```python
from build123d import *

# Parameters (mm, degrees)
SKETCH_1_W          = 220
SKETCH_1_H          = 7
SKETCH_1_R          = 1.6
EXTRUDE_1_DEPTH     = 30
SKETCH_2_W          = 220
SKETCH_2_H          = 5
CUT_EXTRUDE_1_DEPTH = 3
SKETCH_3_W          = 33.308675227
SKETCH_3_H          = 18
SKETCH_3_W_2        = 33.368675227
CUT_EXTRUDE_2_DEPTH = 223.146348158
SKETCH_6_W          = 153.495185447
SKETCH_6_H          = 7
EXTRUDE_2_DEPTH     = 3
SKETCH_7_R          = 1.8
CUT_EXTRUDE_3_DEPTH = 10
CUT_EXTRUDE_START   = -10
SKETCH_8_R          = 1.8
CUT_EXTRUDE_4_DEPTH = 10
CUT_EXTRUDE_5_DEPTH = 223.571336879


with BuildPart() as part:
    # Эскиз1 → Бобышка-Вытянуть1 (new body)
    with BuildSketch(Plane.XY):
        with Locations((110, 3.5)):
            Rectangle(SKETCH_1_W, SKETCH_1_H)
        with Locations((37.97, 3.5)):
            Circle(SKETCH_1_R, mode=Mode.SUBTRACT)
        with Locations((55.97, 3.5)):
            Circle(SKETCH_1_R, mode=Mode.SUBTRACT)
        with Locations((73.97, 3.5)):
            Circle(SKETCH_1_R, mode=Mode.SUBTRACT)
        with Locations((91.97, 3.5)):
            Circle(SKETCH_1_R, mode=Mode.SUBTRACT)
        with Locations((109.97, 3.5)):
            Circle(SKETCH_1_R, mode=Mode.SUBTRACT)
        with Locations((127.97, 3.5)):
            Circle(SKETCH_1_R, mode=Mode.SUBTRACT)
        with Locations((145.97, 3.5)):
            Circle(SKETCH_1_R, mode=Mode.SUBTRACT)
        with Locations((163.97, 3.5)):
            Circle(SKETCH_1_R, mode=Mode.SUBTRACT)
        with Locations((181.97, 3.5)):
            Circle(SKETCH_1_R, mode=Mode.SUBTRACT)
    extrude(amount=EXTRUDE_1_DEPTH)

    # Эскиз2 → Вырез-Вытянуть1 (cut)
    with BuildSketch(Plane(origin=(0, 7, 0), x_dir=(1, 0, 0), z_dir=(0, 1, 0))):
        with Locations((110, -2.5)):
            Rectangle(SKETCH_2_W, SKETCH_2_H)
    extrude(amount=-CUT_EXTRUDE_1_DEPTH, mode=Mode.SUBTRACT)

    # Эскиз3 → Вырез-Вытянуть2 (cut, through all)
    with BuildSketch(Plane(origin=(0, 7, 0), x_dir=(1, 0, 0), z_dir=(0, 1, 0))):
        with Locations((16.654337614, -9)):
            Rectangle(SKETCH_3_W, SKETCH_3_H)
        with Locations((203.315662387, -9)):
            Rectangle(SKETCH_3_W_2, SKETCH_3_H)
    extrude(amount=-CUT_EXTRUDE_2_DEPTH, mode=Mode.SUBTRACT)

    # Эскиз6 → Бобышка-Вытянуть2 (add)
    with BuildSketch(Plane.XY.offset(30)):
        with Locations((109.88373205, 3.5)):
            Rectangle(SKETCH_6_W, SKETCH_6_H)
    extrude(amount=EXTRUDE_2_DEPTH)

    # Эскиз7 → Вырез-Вытянуть3 (cut)
    with BuildSketch(Plane.ZY):
        with Locations((24, 3.5)):
            Circle(SKETCH_7_R)
    extrude(amount=-CUT_EXTRUDE_3_DEPTH, mode=Mode.SUBTRACT)

    # Эскиз8 → Вырез-Вытянуть4 (cut)
    with BuildSketch(Plane(origin=(220, 0, 0), x_dir=(0, 0, -1), z_dir=(1, 0, 0)).offset(CUT_EXTRUDE_START)):
        with Locations(Location((-24, 3.5, 0), (0, 0, 180))):
            Circle(SKETCH_8_R)
    extrude(amount=CUT_EXTRUDE_4_DEPTH, mode=Mode.SUBTRACT)

    # Эскиз9 → Вырез-Вытянуть5 (cut, through all)
    with BuildSketch(Plane(origin=(220, 0, 0), x_dir=(0, 0, -1), z_dir=(1, 0, 0))):
        Polygon((-33, 0), (-33, 3.5), (-25.349385808, 0), align=None)
    extrude(amount=-CUT_EXTRUDE_5_DEPTH, mode=Mode.SUBTRACT)


solid = part.part
```
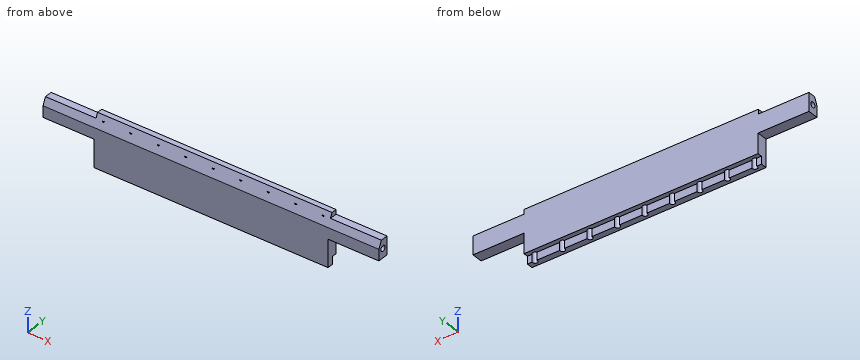
Build history of the part. All positions in model axes, mm. Coordinates: 2 decimals unless noted, no trailing zeros. Order: outer loops, then holes, each group sorted by start corner. A loop starts at its lowest first (then second) coordinate and runs counter-clockwise, first axis right, second up. Notation, with made-up numbers: M -9.5,20.5 L 7.5,20.5 A22 ccw 7.5,57.5 Z; hole C -25,33.25 d9. An arc over 180 degrees is marked long. One line per question, with ' | ' between items. Start each with the question number.
1. Cut at A-A (z = 16). Count the separate pieces of the cut face and the enclosed holes in it, plus the area to 3 significant figures.
2. Wall check: line 1 along Z through (x, y) = (216.5, 3.5); line 2 along Y through (x, z) = (127.97, 15); line 3 along Z through (x, y) = (102, 6). Give the ranges that are in metal, low to high. Write a range as [from, to].
3. Cut at B-B (x = 22.5). Write the cut outline in (y, z), plus the area to 3 significant figures.
4. Flat gauge pins, fed straight in: P1, Ø3, axis at x = 145.97, y = 3.5, coming from the -Z side; P2, Ø3.5, axis at x = 34.5, z = 1.5, coming from the +Y side; P3, Ø1.5, axis at y = 5, z = 31, coming from the -X side. Where does each tip first touch, or does it go through?
5. Cut at C-C (x = 175). Write the cut outline in (y, z), plus the area to 3 significant figures.
The answers:
1) separate pieces: 1 | enclosed holes: 9 | area: 1,000 mm2
2) line 1: z = [18, 22.2], [25.8, 30] | line 2: y = [0, 1.9], [5.1, 7] | line 3: z = [5, 33]
3) outline: M 0,18 L 7,18 L 7,30 L 2.13,30 L 0,25.35 Z | area: 79.1 mm2
4) P1: stops at z = 30 | P2: stops at y = 4 | P3: stops at x = 33.14
5) outline: M 0,0 L 4,0 L 4,5 L 7,5 L 7,33 L 3.5,33 L 0,25.35 Z | area: 203 mm2
